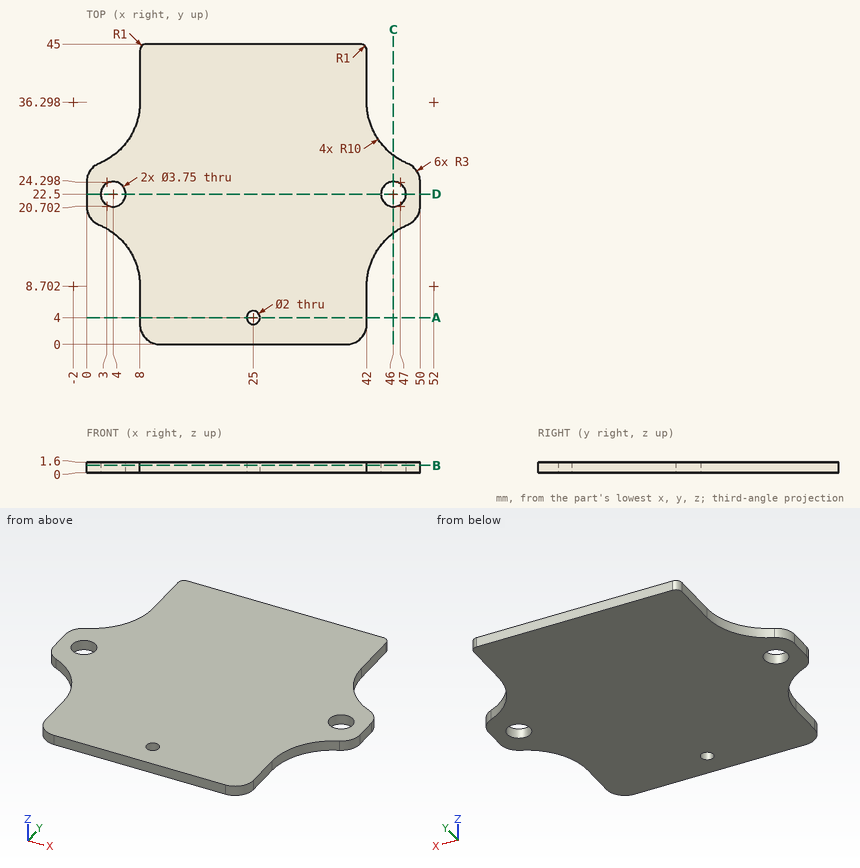
For this review, use the dimensioned drawing (mm, ordinates from the lowest corner) and the shaded views. Coordinates: 2 decimals unless noted, no trailing zeros. Loops run counter-clockwise (first coordinate to the right, second up) from the corner with the lowest first, then second, coordinate; pieces in that order, holes last. Notation, with made-up numbers: (48.5, 16.5) -> (67.5, 16.5) arc R15 cw to (67.5, 36.5) -> close; hole circle Ø4 at (16, 14.25). An arc over 180 degrees is marked (long way). Use a Markdown table: item, result. Add a question column.
1. To check wall thickness, follow line 1 (Y direction, x = 25, z = 0.55); line 2 (X direction, y = 20.5, z = 0.7); line 3 (Y direction, x = 4, z = 1.15) (3 decimals). State the ranges of each line that lie inside material, in increasing order.
2. Add section D-D on y = 22.5. Write out the cut boundary in (x, z) (3 decimals).
3. Add section C-C on x = 46. Write out the cut boundary in (y, z) (3 decimals), plus the area to 3 significant figures.
4. Add section B-B on z = 1.15. Write out the cut boundary in (x, y) (3 decimals).
5. Clearance check with flat-ended pins moving along their axes: pin 1 Ø0.8 at (y, z) = (38.5, 1) entering from +X; pin 2 Ø3 at (x, y) = (46, 22.5) entering from -Z; pin 3 Ø0.8 at (y, z) = (4.5, 0.5) entering from -X. State where each tip first meets the part, or that it passes through.
6. Add section A-A on y = 4. Write out the cut boundary in (x, z).
Returned:
| question | item | result |
|---|---|---|
| 1 | line 1 | y = 0 to 3, 5 to 45 |
| 1 | line 2 | x = 0.01 to 49.99 |
| 1 | line 3 | y = 16.702 to 20.625, 24.375 to 28.298 |
| 2 | outline | (0, 0) -> (2.125, 0) -> (2.125, 1.6) -> (0, 1.6) -> close; (5.875, 0) -> (44.125, 0) -> (44.125, 1.6) -> (5.875, 1.6) -> close; (47.875, 0) -> (50, 0) -> (50, 1.6) -> (47.875, 1.6) -> close |
| 3 | outline | (16.702, 0) -> (20.625, 0) -> (20.625, 1.6) -> (16.702, 1.6) -> close; (24.375, 0) -> (28.298, 0) -> (28.298, 1.6) -> (24.375, 1.6) -> close |
| 3 | area | 12.6 mm² |
| 4 | outline | (0, 20.702) arc R3 ccw to (1.846, 17.933) arc R10 cw to (8, 8.702) -> (8, 3) arc R3 ccw to (11, 0) -> (39, 0) arc R3 ccw to (42, 3) -> (42, 8.702) arc R10 cw to (48.154, 17.933) arc R3 ccw to (50, 20.702) -> (50, 24.298) arc R3 ccw to (48.154, 27.067) arc R10 cw to (42, 36.298) -> (42, 44) arc R1 ccw to (41, 45) -> (9, 45) arc R1 ccw to (8, 44) -> (8, 36.298) arc R10 cw to (1.846, 27.067) arc R3 ccw to (0, 24.298) -> close; hole circle Ø3.75 at (4, 22.5); hole circle Ø2 at (25, 4); hole circle Ø3.75 at (46, 22.5) |
| 5 | pin 1 | stops at x = 42 |
| 5 | pin 2 | passes through |
| 5 | pin 3 | stops at x = 8 |
| 6 | outline | (8, 0) -> (24, 0) -> (24, 1.6) -> (8, 1.6) -> close; (26, 0) -> (42, 0) -> (42, 1.6) -> (26, 1.6) -> close |
